Check sheet for the modelled part. Datum: model origin and axes. Units: mm. Round coordinates to 2 decimals unless told otherwise and drop trailing zeros. Write each loop counter-clockwise with the first axis right and the second up, starting at its lowest first coordinate (ties: lowest second). Pieces come first, ordered by that corner, then holes. Notation, with made-up numbers: (37.25, 51.5) - (89.25, 51.5) arc R11 cw to (89.25, 62.5) - close; hole circle Ø8 at (2.25, -16). An arc over 180 degrees is marked (long way). Answer as a JSON object with one key per item and string values. Group by question number.
Item 1: Sectioned sample at C-C on z = 2.6. Count the separate pieces of the cut face and the enclosed holes in it, plus the area to 3 significant figures.
Item 2: Sectioned sample at B-B on x = 0. Record the boundary of the cut face in (y, z) (1 decimal).
Item 3: Sectioned sample at D-D on y = 7.25. Record the boundary of the cut face in (x, z) (3 decimals).
Item 4: Thickness scan on line 1 (Y direction, x = 63.5, z = 1.15) (1 decimal); line 2 (X direction, y = -0.5, z = 2.1); line 3 (X direction, y = 3, z = 1.4). Record the ranges inside material, lowest first.
Item 5: Sectioned sample at A-A on y = 0. Record the boundary of the cut face in (x, z) (1 decimal).
```python
from build123d import *

# Parameters (mm, degrees)
F0_R     = 1.5875
F1_DEPTH = 3.175


with BuildPart() as f1:
    # F0 (on Top) → F1 (new body)
    with BuildSketch(Plane.XY):
        with BuildLine():
            ThreePointArc((63.5, -9.525), (73.025, 0), (63.5, 9.525))
            Line((63.5, 9.525), (-63.5, 9.525))
            ThreePointArc((-63.5, 9.525), (-73.025, 0), (-63.5, -9.525))
            Line((-63.5, -9.525), (63.5, -9.525))
        make_face()
        with Locations((-63.5, 0)):
            Circle(F0_R, mode=Mode.SUBTRACT)
        Circle(F0_R, mode=Mode.SUBTRACT)
        with Locations((63.5, 0)):
            Circle(F0_R, mode=Mode.SUBTRACT)
    extrude(amount=F1_DEPTH)


solid = f1.part
```
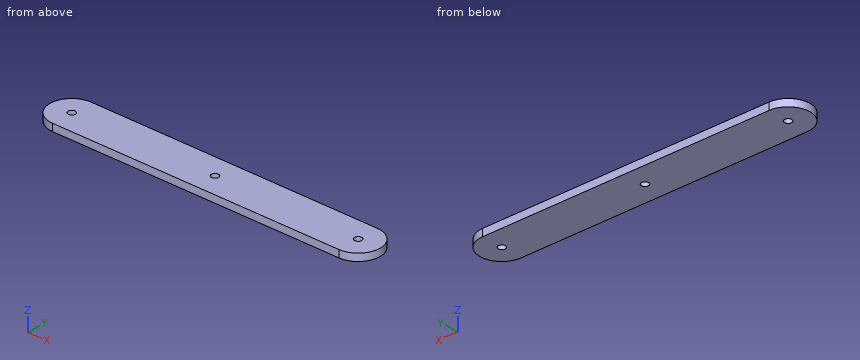
Completed:
{
 "1": {"separate pieces": "1", "enclosed holes": "3", "area": "2,680 mm²"},
 "2": {"outline": "(-9.5, 0) - (-1.6, 0) - (-1.6, 3.2) - (-9.5, 3.2) - close; (1.6, 0) - (9.5, 0) - (9.5, 3.2) - (1.6, 3.2) - close"},
 "3": {"outline": "(-69.678, 0) - (69.678, 0) - (69.678, 3.175) - (-69.678, 3.175) - close"},
 "4": {"line 1": "-9.5 to -1.6, 1.6 to 9.5", "line 2": "-73.01 to -65.01, -61.99 to -1.51, 1.51 to 61.99, 65.01 to 73.01", "line 3": "-72.54 to 72.54"},
 "5": {"outline": "(-73, 0) - (-65.1, 0) - (-65.1, 3.2) - (-73, 3.2) - close; (-61.9, 0) - (-1.6, 0) - (-1.6, 3.2) - (-61.9, 3.2) - close; (1.6, 0) - (61.9, 0) - (61.9, 3.2) - (1.6, 3.2) - close; (65.1, 0) - (73, 0) - (73, 3.2) - (65.1, 3.2) - close"}
}
